from build123d import *

# Parameters (mm, degrees)
SCHIZZO1_R                       = 50
SCHIZZO1_R_2                     = 4
ESTRUSIONE_ESTRUSIONE1_DEPTH     = 10
SCHIZZO2_R                       = 15
ESTRUSIONE_ESTRUSIONE2_DEPTH     = 10
FORO_FILETTATO_M24_1_D           = 21
FORO_FILETTATO_M24_1_CSINK_D     = 24.05
FORO_FILETTATO_M24_1_CSINK_ANGLE = 120
SMUSSO1_SIZE                     = 2


with BuildPart() as part:
    # Schizzo1 → Estrusione-Estrusione1 (new body)
    with BuildSketch(Plane.XY):
        Circle(SCHIZZO1_R)
        with Locations((0, 26.870057685)):
            Circle(SCHIZZO1_R_2, mode=Mode.SUBTRACT)
        with Locations((26.870057685, 0)):
            Circle(SCHIZZO1_R_2, mode=Mode.SUBTRACT)
        with Locations((0, -26.870057685)):
            Circle(SCHIZZO1_R_2, mode=Mode.SUBTRACT)
        with Locations((-26.870057685, 0)):
            Circle(SCHIZZO1_R_2, mode=Mode.SUBTRACT)
    extrude(amount=ESTRUSIONE_ESTRUSIONE1_DEPTH)

    # Schizzo2 → Estrusione-Estrusione2 (add)
    with BuildSketch(Plane.XY.offset(10)):
        Circle(SCHIZZO2_R)
    extrude(amount=ESTRUSIONE_ESTRUSIONE2_DEPTH)

    # Foro filettato M24-1 (through all)
    with Locations(Plane(origin=(0, 0, 0), x_dir=(-1, 0, 0), z_dir=(0, 0, -1))):
        with Locations((0, 0)):
            CounterSinkHole(FORO_FILETTATO_M24_1_D / 2, FORO_FILETTATO_M24_1_CSINK_D / 2, counter_sink_angle=FORO_FILETTATO_M24_1_CSINK_ANGLE)

    # Smusso1
    smusso1_edges = [part.edges().sort_by_distance(p)[0] for p in [
        (-10.5, 0, 20),
    ]]
    chamfer(smusso1_edges, length=SMUSSO1_SIZE)


solid = part.part
For this review, take the finished solid that the model builds, in its own axes (mm). A direction names the side the tool comes from. Coordinates: 2 decimals unless noted, no trailing zeros. Loops run counter-clockwise (first coordinate to the right, second up) from the corner with the lowest first, then second, coordinate; pieces in that order, holes last. Notation, with made-up numbers: (46, -10) - (101, -10) arc R14 ccw to (101, 3) - close; hole circle Ø1 at (40.5, 17). An arc over 180 degrees is marked (long way). Return JSON: item names as keys, results as strings.
Item 1: Mouldability with a two-part tool opening along Y and no side actions: class faces 3 (the cylindrical face through (47.69, 15.02, 4.93)), 4 (the flat face through (-12, -10, 10)), 5 (the cylindrical face through (30.685, 1.201, 4.93)) as pulls with the +Y half, pulls with the -Y half, needs draft (parallel to the pull), parting line crosses it, or undercut.
Determined:
{"face 3": "parting line crosses it", "face 4": "needs draft", "face 5": "undercut"}
Item 2: Take a section at D-D (x = -27.5). Give the boundary of the cut face in (y, z), then the cut area to 3 significant figures.
Determined:
{"outline": "(-41.76, 0) - (-3.95, 0) - (-3.95, 10) - (-41.76, 10) - close; (3.95, 0) - (41.76, 0) - (41.76, 10) - (3.95, 10) - close", "area": "756 mm2"}
Item 3: For line 1 (Y direction, x = 0, z = 7); line 2 (X direction, y = -2, z = 8.25); line 3 (Y direction, x = 0, z = 13), list the stretches that pass through material, from the lowest coordinate up.
Determined:
{"line 1": "y = -50 to -30.87, -22.87 to -10.5, 10.5 to 22.87, 30.87 to 50", "line 2": "x = -49.96 to -30.33, -23.41 to -10.31, 10.31 to 23.41, 30.33 to 49.96", "line 3": "y = -15 to -10.5, 10.5 to 15"}
Item 4: Take a section at A-A (y = 0). Give the boundary of the cut face in (x, z) (3 decimals).
Determined:
{"outline": "(-50, 0) - (-30.87, 0) - (-30.87, 10) - (-50, 10) - close; (-22.87, 0) - (-12.025, 0) - (-10.5, 0.88) - (-10.5, 18) - (-12.5, 20) - (-15, 20) - (-15, 10) - (-22.87, 10) - close; (10.5, 0.88) - (12.025, 0) - (22.87, 0) - (22.87, 10) - (15, 10) - (15, 20) - (12.5, 20) - (10.5, 18) - close; (30.87, 0) - (50, 0) - (50, 10) - (30.87, 10) - close"}
Item 5: For faces 1 (the cylindrical face through (-14.985, 0.66, 14.93)), 2 (the cylindrical face through (-0.521, 30.836, 4.93)), list the 3-axis set-ups (+Z, -Z, +X, -X, +Y, -Y) from which the entire face can be reached by the end or side of a thin tool; tool diameter is ignored.
Determined:
{"face 1": "+Z", "face 2": "+Z, -Z"}
Item 6: Take a section at C-C (y = -25). Give the boundary of the cut face in (x, z).
Determined:
{"outline": "(-43.3, 0) - (-3.54, 0) - (-3.54, 10) - (-43.3, 10) - close; (3.54, 0) - (43.3, 0) - (43.3, 10) - (3.54, 10) - close"}
Item 7: Insertion check: pin 1 (6 mm diameter, centred on y = 26, z = 4.5, fed in from +X); pin 2 (6.5 mm diameter, centred on x = 26.87, y = 0, fed in from -Z); pin 3 (2 mm diameter, centred on x = 24, y = 26.5, fed in from +Z); pin 4 (12 mm diameter, centred on x = -19, z = 15, fed in from -Y). Each pin has a flat end and moves straight along its axis. Give the tip position at first contact, or say it passes through.
Determined:
{"pin 1": "stops at x = 44.4", "pin 2": "passes through", "pin 3": "stops at z = 10", "pin 4": "stops at y = -47.48"}
